```python
from build123d import *

# Parameters (mm, degrees)
BOSS_EXTRUDE1_DEPTH = 32
SKETCH2_R           = 1.05
CUT_EXTRUDE1_DEPTH  = 32
SKETCH3_R           = 1.05
CUT_EXTRUDE2_DEPTH  = 32


with BuildPart() as part:
    # Sketch1 → Boss-Extrude1 (new body)
    with BuildSketch(Plane(origin=(0, 0, 0), x_dir=(1, 0, 0), z_dir=(0, 1, 0))):
        Polygon((-16, 11.757359313), (0, -4.242640687), (16, 11.757359313), (13.878679656, 13.878679656), (0, 0), (-13.878679656, 13.878679656), align=None)
    extrude(amount=BOSS_EXTRUDE1_DEPTH)

    # Sketch2 → Cut-Extrude1 (cut)
    with BuildSketch(Plane(origin=(0, 0, 0), x_dir=(-0.7071067811865538, 0, -0.7071067811865414), z_dir=(0.7071067811865414, 0, -0.7071067811865538))):
        with Locations((17.677416998, 16)):
            Circle(SKETCH2_R)
    extrude(amount=-CUT_EXTRUDE1_DEPTH, mode=Mode.SUBTRACT)

    # Sketch3 → Cut-Extrude2 (cut)
    with BuildSketch(Plane(origin=(0, 0, 0), x_dir=(-0.7071067811865475, 0, 0.7071067811865477), z_dir=(-0.7071067811865477, 0, -0.7071067811865475))):
        with Locations((-17.677416998, 16)):
            Circle(SKETCH3_R)
    extrude(amount=-CUT_EXTRUDE2_DEPTH, mode=Mode.SUBTRACT)


solid = part.part
```
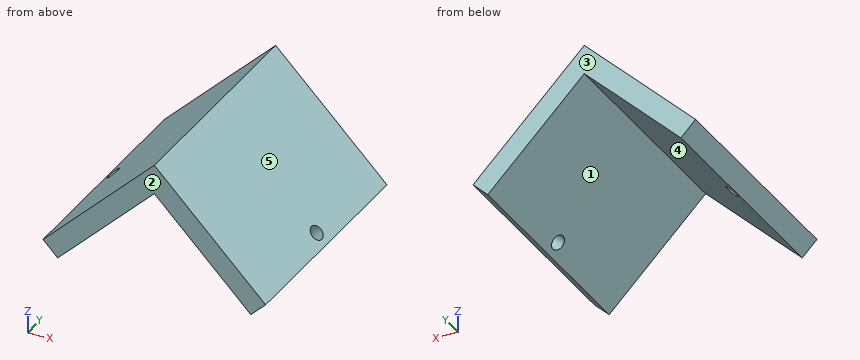
CAD build for the part. Positions are in the model's coordinates, mm. Face numbers are marked on the shaded views. A direction names the side the tool comes from. Give positions to 0.01 mm unless a question says otherwise; leave off trailing zeros. Write each loop counter-clockwise with the first axis right and the second up, starting at its lowest first coordinate (ties: lowest second). Pieces come first, ordered by that corner, then holes. Notation, with made-up numbers: M 75.5,69 L 99.5,69 A22 ccw 99.5,83 Z; hole C 37.5,37 d11. An arc over 180 degrees is marked long. Return JSON: item names as keys, results as strings. Group by question number.
(1) Band-saw the part on B-B (y = 27). Give the cut face in (x, z), and give its area (3 significant figures).
(2) 3-axis set-ups, long thin cutter, end or side, ignore diameter. For the marked faces 1 and 2: which of +Z, -Z, +X, -X, +Y, -Y reach the whole face in a straight line?
(3) Band-saw the part on C-C (x = 2). Give the cut face in (y, z), and give its area (3 significant figures).
(4) Drill centre lines: L1, parallel to X at y = 24.5, z = -12; L2, parallel to X at y = 5.5, z = -9.75; L3, parallel to Z at x = 9.5, y = 22.5. Where is each one in solid material? Low to high. Write a range as [from, to].
(5) Mould opens along X. For the marked faces 3, 4 and 5 say: pulls with the +X half, pulls with the -X half, needs draft (parallel to the pull), parting line crosses it, or undercut.
(6) Flat gauge pins, fed straight in: pin 1 Ø4 at (x, y) = (-3.5, 8.5) entering from +Z; pin 2 Ø6 at (x, z) = (-9, -10) entering from +Y; pin 3 Ø10 at (y, z) = (22.5, -2.5) entering from -X; pin 4 Ø1 at (y, z) = (23, -2) entering from -X. Where does each tip first touch, or does it go through?
(7) Band-saw the part on A-A (z = -0.75). Give the cut face in (x, y), and give its area (3 significant figures).
Entries:
{
 "1": {"outline": "M -16,-11.76 L -13.88,-13.88 L 0,0 L 13.88,-13.88 L 16,-11.76 L 0,4.24 Z", "area": "127 mm^2"},
 "2": {"face 1": "-Z, +Y, -Y", "face 2": "+Z, -Z, +X, -X, -Y"},
 "3": {"outline": "M 0,-2 L 32,-2 L 32,2.24 L 0,2.24 Z", "area": "136 mm^2"},
 "4": {"L1": "x = [-15.76, -12], [12, 15.76]", "L2": "x = [-13.99, -9.75], [9.75, 13.99]", "L3": "z = [-9.5, -5.26]"},
 "5": {"face 3": "needs draft", "face 4": "undercut", "face 5": "pulls with the +X half"},
 "6": {"pin 1": "stops at z = 2.74", "pin 2": "stops at y = 32", "pin 3": "stops at x = -11.74", "pin 4": "stops at x = -6.74"},
 "7": {"outline": "M -4.99,0 L -0.75,0 L -0.75,32 L -4.99,32 Z; M 0.75,0 L 4.99,0 L 4.99,32 L 0.75,32 Z", "area": "272 mm^2"}
}
